Model file for the job. Use its own axes, mm. A direction names the side the tool comes from. Coordinates: 2 decimals unless noted, no trailing zeros. Order: outer loops, then holes, each group sorted by start corner. A loop starts at its lowest first (then second) coordinate and runs counter-clockwise, first axis right, second up. Notation, with made-up numbers: (28, 60.5) -> (77, 60.5) arc R33 cw to (77, 88.5) -> close; hole circle Ø7 at (-19.5, 19). An arc over 180 degrees is marked (long way). Return JSON: item names as keys, results as strings. Group by question number.
1) Flat gauge pins, fed straight in: pin 1 (18 mm diameter, centred on x = -4, z = 4.5, fed in from +Y); pin 2 (4 mm diameter, centred on x = -6, y = 8.5, fed in from +Z); pin 3 (3 mm diameter, centred on x = -13.5, z = 13.5, fed in from +Y); pin 4 (3 mm diameter, centred on x = 7.5, y = 12, fed in from -Z). Where does each tip first touch, or does it go through?
2) Cut at C-C (x = -13.5). State how many separate pieces and enclosed holes the cut face has, and give its area (3 significant figures).
3) Cut at A-A (z = 0). Write the cut outline in (x, y).
4) Which spindle directions (+Z, -Z, +X, -X, +Y, -Y) get a long thin tool onto all of the face, cutting with end or side? Do faces 4 (the flat face through (-17.5, 2, 0)), 5 (the flat face through (5, 10, 0)), 6 (the flat face through (10, 9, -4)). Say none if no direction does.
5) Pull direction Z, two halves, no side cores. Call faces 1 (the cylindrical face through (5.19, 12.96, 9.98)), 2 (the flat face through (8, 4, -8)), 3 (the cylindrical face through (-16.93, 2.03, -16.9)): +Z half, -Z half, draft (parallel to the pull), parting line (faces both ways), or undercut.
6) Probe line 1 (X direction, y = 2.15, z = -13.5); line 2 (Z direction, x = 0, y = 13.75). List the from-to ranges inside material, lowest first.
7) Cut at B-B (y = 1). Write the cut outline in (x, z), and give its area (3 significant figures).
from build123d import *

# Parameters (mm, degrees)
CROQUIS1_W              = 35
CROQUIS1_H              = 35
CROQUIS1_R              = 1.65
CROQUIS1_R_2            = 9
SALIENTE_EXTRUIR1_DEPTH = 4
REDONDEO2_R             = 2
CROQUIS1_8_R            = 9
CROQUIS1_8_R_2          = 4.05
SALIENTE_EXTRUIR2_DEPTH = 9
CROQUIS2_R              = 16.5
CROQUIS2_R_2            = 11.25
SALIENTE_EXTRUIR3_DEPTH = 7
REDONDEO3_R             = 1.5
CROQUIS2_3_R            = 11.25
CROQUIS2_3_R_2          = 9
CROQUIS2_3_R_3          = 4.05
SALIENTE_EXTRUIR4_DEPTH = 1
REDONDEO4_R             = 1.5
REDONDEO5_R             = 1


with BuildPart() as part:
    # Croquis1 → Saliente-Extruir1 (new body)
    with BuildSketch(Plane(origin=(0, 0, 0), x_dir=(1, 0, 0), z_dir=(0, 1, 0))):
        Rectangle(CROQUIS1_W, CROQUIS1_H)
        with Locations((-13.5, -13.5)):
            Circle(CROQUIS1_R, mode=Mode.SUBTRACT)
        with Locations((13.5, -13.5)):
            Circle(CROQUIS1_R, mode=Mode.SUBTRACT)
        with Locations((13.5, 13.5)):
            Circle(CROQUIS1_R, mode=Mode.SUBTRACT)
        with Locations((-13.5, 13.5)):
            Circle(CROQUIS1_R, mode=Mode.SUBTRACT)
        Circle(CROQUIS1_R_2, mode=Mode.SUBTRACT)
    extrude(amount=SALIENTE_EXTRUIR1_DEPTH)

    # Redondeo2
    redondeo2_edges = [part.edges().sort_by_distance(p)[0] for p in [
        (17.5, 2, 17.5),
        (-17.5, 2, 17.5),
        (-17.5, 2, -17.5),
        (17.5, 2, -17.5),
    ]]
    fillet(redondeo2_edges, radius=REDONDEO2_R)

    # Croquis1<8> → Saliente-Extruir2 (add)
    with BuildSketch(Plane(origin=(0, 0, 0), x_dir=(1, 0, 0), z_dir=(0, 1, 0))):
        Circle(CROQUIS1_8_R)
        Circle(CROQUIS1_8_R_2, mode=Mode.SUBTRACT)
    extrude(amount=SALIENTE_EXTRUIR2_DEPTH)

    # Redondeo3
    redondeo3_edges = [part.edges().sort_by_distance(p)[0] for p in [
        (-9, 4, 0),
    ]]
    fillet(redondeo3_edges, radius=REDONDEO3_R)



with BuildPart() as body_2:
    # Croquis2 → Saliente-Extruir3 (new body)
    with BuildSketch(Plane(origin=(0, 9, 0), x_dir=(1, 0, 0), z_dir=(0, 1, 0))):
        Circle(CROQUIS2_R)
        Circle(CROQUIS2_R_2, mode=Mode.SUBTRACT)
    extrude(amount=SALIENTE_EXTRUIR3_DEPTH)


with BuildPart() as part_1:
    add(part.part)

    add(body_2.part)  # Saliente-Extruir4 merges body 2
    # Croquis2<3> → Saliente-Extruir4 (add)
    with BuildSketch(Plane(origin=(0, 9, 0), x_dir=(1, 0, 0), z_dir=(0, 1, 0))):
        Circle(CROQUIS2_3_R)
        Circle(CROQUIS2_3_R_2, mode=Mode.SUBTRACT)
        Circle(CROQUIS2_3_R_2)
        Circle(CROQUIS2_3_R_3, mode=Mode.SUBTRACT)
    extrude(amount=SALIENTE_EXTRUIR4_DEPTH)

    # Redondeo4
    redondeo4_edges = [part_1.edges().sort_by_distance(p)[0] for p in [
        (-9, 9, 0),
    ]]
    fillet(redondeo4_edges, radius=REDONDEO4_R)

    # Redondeo5
    redondeo5_edges = [part_1.edges().sort_by_distance(p)[0] for p in [
        (-16.5, 9, 0),
    ]]
    fillet(redondeo5_edges, radius=REDONDEO5_R)


solid = part_1.part
Answers below:
{
 "1": {"pin 1": "stops at y = 16", "pin 2": "stops at z = 15.86", "pin 3": "passes through", "pin 4": "stops at z = -15.37"},
 "2": {"separate pieces": "4", "enclosed holes": "0", "area": "246 mm^2"},
 "3": {"outline": "(-17.5, 0) -> (-4.05, 0) -> (-4.05, 10) -> (-11.25, 10) -> (-11.25, 16) -> (-16.5, 16) -> (-16.5, 10) arc R1 ccw to (-15.5, 9) -> (-10.5, 9) arc R1.5 cw to (-9, 7.5) -> (-9, 5.5) arc R1.5 cw to (-10.5, 4) -> (-17.5, 4) -> close; (4.05, 0) -> (17.5, 0) -> (17.5, 4) -> (10.5, 4) arc R1.5 cw to (9, 5.5) -> (9, 7.5) arc R1.5 cw to (10.5, 9) -> (15.5, 9) arc R1 ccw to (16.5, 10) -> (16.5, 16) -> (11.25, 16) -> (11.25, 10) -> (4.05, 10) -> close"},
 "4": {"face 4": "+Z, -Z, -X, +Y, -Y", "face 5": "+Y", "face 6": "none"},
 "5": {"face 1": "undercut", "face 2": "draft", "face 3": "-Z half"},
 "6": {"line 1": "x = -17.5 to -15.15, -11.85 to 11.85, 15.15 to 17.5", "line 2": "z = -16.5 to -11.25, 11.25 to 16.5"},
 "7": {"outline": "(-17.5, -15.5) arc R2 ccw to (-15.5, -17.5) -> (15.5, -17.5) arc R2 ccw to (17.5, -15.5) -> (17.5, 15.5) arc R2 ccw to (15.5, 17.5) -> (-15.5, 17.5) arc R2 ccw to (-17.5, 15.5) -> close; hole circle Ø3.3 at (-13.5, -13.5); hole circle Ø3.3 at (-13.5, 13.5); hole circle Ø8.1 at (0, 0); hole circle Ø3.3 at (13.5, -13.5); hole circle Ø3.3 at (13.5, 13.5)", "area": "1,140 mm^2"}
}
